Design review of the part built by this model. Coordinates are the model's own, in mm. A direction names the side the tool comes from. Round coordinates to 2 decimals unless told otherwise and drop trailing zeros. Loops run counter-clockwise (first coordinate to the right, second up) from the corner with the lowest first, then second, coordinate; pieces in that order, holes last. Notation, with made-up numbers: M -39,83.5 L -11,83.5 A21 cw -11,91.5 Z; hole C -20.75,55.25 d8. An arc over 180 degrees is marked long. Use a Markdown table: item, result.
from build123d import *

# Parameters (mm, degrees)
F1_DEPTH = 3
F2_DEPTH = 10
F3_R     = 4
F4_R     = 0.5


with BuildPart() as f1:
    # F0 (on Top) → F1 (new body)
    with BuildSketch(Plane.XY):
        Polygon((-10.9281279506, 21.8490213156), (-10.9281279506, -20.5509786844), (4.2718720494, -20.5509786844), (4.2718720494, 6.6490213156), (31.4718720494, 6.6490213156), (31.4718720494, 21.8490213156), align=None)
        Polygon((28.4718720494, 18.8490213156), (28.4718720494, 9.6490213156), (1.2718720494, 9.6490213156), (1.2718720494, -17.5509786844), (-7.9281279506, -17.5509786844), (-7.9281279506, 18.8490213156), align=None, mode=Mode.SUBTRACT)
        Polygon((1.2718720494, 9.6490213156), (28.4718720494, 9.6490213156), (28.4718720494, 18.8490213156), (-7.9281279506, 18.8490213156), (-7.9281279506, -17.5509786844), (1.2718720494, -17.5509786844), align=None)
        Polygon((-1.7281279506, -14.5509786844), (-4.9281279506, -14.5509786844), (-4.9281279506, 15.8490213156), (25.4718720494, 15.8490213156), (25.4718720494, 12.6490213156), (-1.7281279506, 12.6490213156), align=None, mode=Mode.SUBTRACT)
        Polygon((-4.9281279506, 15.8490213156), (-4.9281279506, -14.5509786844), (-1.7281279506, -14.5509786844), (-1.7281279506, 12.6490213156), (25.4718720494, 12.6490213156), (25.4718720494, 15.8490213156), align=None)
    extrude(amount=F1_DEPTH)

    # F0 (on Top) → F2 (join)
    with BuildSketch(Plane.XY):
        Polygon((1.2718720494, 9.6490213156), (28.4718720494, 9.6490213156), (28.4718720494, 18.8490213156), (-7.9281279506, 18.8490213156), (-7.9281279506, -17.5509786844), (1.2718720494, -17.5509786844), align=None)
        Polygon((-1.7281279506, -14.5509786844), (-4.9281279506, -14.5509786844), (-4.9281279506, 15.8490213156), (25.4718720494, 15.8490213156), (25.4718720494, 12.6490213156), (-1.7281279506, 12.6490213156), align=None, mode=Mode.SUBTRACT)
    extrude(amount=F2_DEPTH)

    # F3
    f3_edges = [f1.edges().sort_by_distance(p)[0] for p in [
        (4.271872, -20.550979, 1.5),
        (31.471872, 6.649021, 1.5),
        (31.471872, 21.849021, 1.5),
        (-10.928128, 21.849021, 1.5),
        (-10.928128, -20.550979, 1.5),
        (1.271872, -17.550979, 6.5),
        (28.471872, 9.649021, 6.5),
        (28.471872, 18.849021, 6.5),
        (-7.928128, -17.550979, 6.5),
        (-1.728128, 12.649021, 6.5),
        (-7.928128, 18.849021, 6.5),
    ]]
    fillet(f3_edges, radius=F3_R)

    # F4
    f4_edges = [f1.edges().sort_by_distance(p)[0] for p in [
        (-10.928128, 0.649021, 3),
        (-9.756555, 20.677448, 3),
        (-9.756555, -19.379406, 3),
        (10.271872, 21.849021, 3),
        (-3.328128, -20.550979, 3),
        (30.300299, 20.677448, 3),
        (3.100299, -19.379406, 3),
        (31.471872, 14.249021, 3),
        (4.271872, -4.950979, 3),
        (30.300299, 7.820594, 3),
        (15.871872, 6.649021, 3),
        (1.271872, -1.950979, 3),
        (0.100299, -16.379406, 3),
        (12.871872, 9.649021, 3),
        (-3.328128, -17.550979, 3),
        (27.300299, 10.820594, 3),
        (-6.756555, -16.379406, 3),
        (28.471872, 14.249021, 3),
        (-7.928128, 0.649021, 3),
        (27.300299, 17.677448, 3),
        (-6.756555, 17.677448, 3),
        (10.271872, 18.849021, 3),
        (-7.928128, 0.649021, 10),
        (-6.756555, 17.677448, 10),
        (10.271872, 18.849021, 10),
        (27.300299, 17.677448, 10),
    ]]
    fillet(f4_edges, radius=F4_R)


solid = f1.part
1. Machinability: for faces 1 (the face through (3, 5, 3)), 2 (the face through (1.272, -2, 6)), 3 (the face through (16, 6.649, 1)), which of the approach directions +Z, -Z, +X, -X, +Y, -Y give a long, thin tool a straight path to every point of the face, cutting with its end or side? Answer none if there is none.
Check values:
| item | result |
|---|---|
| face 1 | +Z |
| face 2 | +Z, +X, -Y |
| face 3 | +Z, -Z, +X, -Y |
2. Take a section at B-B on y = 3.5. Give the boundary of the cut face in (x, z), and give its area (3 significant figures).
Check values:
| item | result |
|---|---|
| outline | M -10.93,0 L 4.27,0 L 4.27,2.5 A0.5 ccw 3.77,3 L 1.77,3 A0.5 cw 1.27,3.5 L 1.27,9.5 A0.5 ccw 0.77,10 L -1.73,10 L -1.73,3 L -4.93,3 L -4.93,10 L -7.43,10 A0.5 ccw -7.93,9.5 L -7.93,3.5 A0.5 cw -8.43,3 L -10.43,3 A0.5 ccw -10.93,2.5 Z |
| area | 87.5 mm² |
3. Insertion check: pin 1 (3.5 mm diameter, centred on y = -3, z = 6, fed in from -X); pin 2 (1.3 mm diameter, centred on x = -3.5, z = 6, fed in from -Y); pin 3 (0.6 mm diameter, centred on y = 14.5, z = 6.5, fed in from +X); pin 4 (6 mm diameter, centred on x = 8, y = -15, fed in from +Z). Each pin has a flat end and moves straight along its axis. Give the tip position at first contact, or say it passes through.
Check values:
| item | result |
|---|---|
| pin 1 | stops at x = -7.93 |
| pin 2 | stops at y = -17.55 |
| pin 3 | stops at x = 28.47 |
| pin 4 | passes through |
4. Take a section at D-D on x = 23.5. Give the boundary of the cut face in (y, z), and give its area (3 significant figures).
Check values:
| item | result |
|---|---|
| outline | M 6.65,0 L 21.85,0 L 21.85,2.5 A0.5 ccw 21.35,3 L 19.35,3 A0.5 cw 18.85,3.5 L 18.85,9.5 A0.5 ccw 18.35,10 L 15.85,10 L 15.85,3 L 12.65,3 L 12.65,10 L 10.15,10 A0.5 ccw 9.65,9.5 L 9.65,3.5 A0.5 cw 9.15,3 L 7.15,3 A0.5 ccw 6.65,2.5 Z |
| area | 87.5 mm² |
5. Wall thickness on line 1 along Y through (x, z) = (10.5, 4.5); line 2 along X through (y, z) = (5.5, 4.75); line 3 along Y through (x, z) = (16.5, 0.75): over which ranges is each line inside the solid? List them lowest first. Write a range as from..to.
Check values:
| item | result |
|---|---|
| line 1 | y = 9.65..12.65, 15.85..18.85 |
| line 2 | x = -7.93..-4.93, -1.73..1.27 |
| line 3 | y = 6.65..21.85 |
6. Take a section at C-C on z = 1. Give the boundary of the cut face in (x, y).
Check values:
| item | result |
|---|---|
| outline | M -10.93,-16.55 A4 ccw -6.93,-20.55 L 0.27,-20.55 A4 ccw 4.27,-16.55 L 4.27,6.65 L 27.47,6.65 A4 ccw 31.47,10.65 L 31.47,17.85 A4 ccw 27.47,21.85 L -6.93,21.85 A4 ccw -10.93,17.85 Z |
7. The part is to be moulded in two halves that separate along Y. For faces 4 (the face through (0.07, -16.41, 6.54)), 5 (the face through (25.472, 14, 6)), 6 (the face through (4.272, -5, 1)), say which applies: pulls with the +Y half, pulls with the -Y half, needs draft (parallel to the pull), parting line crosses it, or undercut.
Check values:
| item | result |
|---|---|
| face 4 | pulls with the -Y half |
| face 5 | undercut |
| face 6 | needs draft |
8. Take a section at A-A on z = 6.25. Give the boundary of the cut face in (x, y).
Check values:
| item | result |
|---|---|
| outline | M -7.93,-13.55 A4 ccw -3.93,-17.55 L -2.73,-17.55 A4 ccw 1.27,-13.55 L 1.27,9.65 L 24.47,9.65 A4 ccw 28.47,13.65 L 28.47,14.85 A4 ccw 24.47,18.85 L -3.93,18.85 A4 ccw -7.93,14.85 Z; hole M -4.93,-14.55 L -1.73,-14.55 L -1.73,8.65 A4 cw 2.27,12.65 L 25.47,12.65 L 25.47,15.85 L -4.93,15.85 Z |
